Design review of the part built by this model. Coordinates are the model's own, in mm. Give positions to 0.01 mm unless a question says otherwise; leave off trailing zeros. Loops run counter-clockwise (first coordinate to the right, second up) from the corner with the lowest first, then second, coordinate; pieces in that order, holes last.
from build123d import *

# Parameters (mm, degrees)
F0_R     = 75
F2_DEPTH = 200
F3_R     = 74
F4_DEPTH = 200
F5_DEPTH = 200


with BuildPart() as f2:
    # F0 (on Top) → F2 (new body)
    with BuildSketch(Plane.XY):
        Circle(F0_R)
    extrude(amount=F2_DEPTH)

    # F3 (on face) → F4 (cut)
    with BuildSketch(Plane.XY.offset(200)):
        Circle(F3_R)
    extrude(amount=-F4_DEPTH, mode=Mode.SUBTRACT)

    # F1 (on face) → F5 (cut)
    with BuildSketch(Plane.XY):
        with BuildLine():
            ThreePointArc((15.375163, 73.407114), (0.373019, 74.999072), (-14.644218, 73.55642))
            Line((-14.644218, 73.55642), (-14.644218, 72.327003))
            Line((-14.644218, 72.327003), (15.387964, 72.327003))
            Line((15.387964, 72.327003), (15.375163, 73.407114))
        make_face()
    extrude(amount=-F5_DEPTH, mode=Mode.SUBTRACT)


solid = f2.part
Q1. Take a section at A-A (x = 0). Give the boundary of the cut face in (y, z), plus the area to 3 significant figures.
Results:
outline: (-75, 0) - (-74, 0) - (-74, 200) - (-75, 200) - close; (74, 0) - (75, 0) - (75, 200) - (74, 200) - close
area: 400 mm2
Q2. Wall thickness on line 1 (Y direction, x = 0, z = 65); line 2 (X direction, y = 1.5, z = 178.5) (3 decimals); line 3 (Y direction, x = -30.5, z = 113.5): over which ranges is each line inside the solid? List them lowest first.
Results:
line 1: y = -75 to -74, 74 to 75
line 2: x = -74.985 to -73.985, 73.985 to 74.985
line 3: y = -68.52 to -67.42, 67.42 to 68.52
Q3. Insertion check: pin 1 (4 mm diameter, centred on x = 1, z = 29, fed in from -Y); pin 2 (5 mm diameter, centred on x = -6, z = 98.5, fed in from -Y); pin 3 (12 mm diameter, centred on y = -12, z = 125.5, fed in from +X). Each pin has a flat end and moves straight along its axis. Give the tip position at first contact, or say it passes through.
Results:
pin 1: stops at y = -75
pin 2: stops at y = -74.92
pin 3: stops at x = 74.76
Q4. Draft analysis for pull direction X (two halves, no side actions). For faces 1 (the face through (50, -55, 0)), 2 (the face through (-9.764, 74.362, 98.6)), 3 (the face through (-16.04, -72.24, 101.4)), state which applies: pulls with the +X half, pulls with the -X half, needs draft (parallel to the pull), parting line crosses it, or undercut.
Results:
face 1: needs draft
face 2: parting line crosses it
face 3: undercut
Q5. Take a section at C-C (z = 74.5). Give the boundary of the cut face in (x, y).
Results:
outline: circle Ø150 at (0, 0); hole circle Ø148 at (0, 0)
